Read the model definition and answer for the solid it produces. Units are mm, in the model's axes. Give positions to 0.01 mm unless a question says otherwise; leave off trailing zeros. Order: outer loops, then holes, each group sorted by start corner. A loop starts at its lowest first (then second) coordinate and runs counter-clockwise, first axis right, second up.
```python
from build123d import *

# Parameters (mm, degrees)
SKETCH1_R           = 80.645
BOSS_EXTRUDE1_DEPTH = 7.9375
SKETCH3_R           = 31.877
CUT_EXTRUDE1_DEPTH  = 16.875
CHAMFER1_SIZE       = 3.175
SKETCH5_R           = 5.7546875
CUT_EXTRUDE2_DEPTH  = 16.875
CIRPATTERN1_COUNT   = 5
SKETCH6_R           = 5.7546875
CUT_EXTRUDE3_DEPTH  = 16.875
CIRPATTERN2_COUNT   = 5


with BuildPart() as part:
    # Sketch1 → Boss-Extrude1 (new body, symmetric)
    with BuildSketch(Plane(origin=(0, 0, 0), x_dir=(0, 0, -1), z_dir=(1, 0, 0))):
        Circle(SKETCH1_R)
    extrude(amount=BOSS_EXTRUDE1_DEPTH, both=True)

    # Sketch3 → Cut-Extrude1 (cut, through all)
    with BuildSketch(Plane(origin=(7.9375, 0, 0), x_dir=(0, 0, -1), z_dir=(1, 0, 0))):
        Circle(SKETCH3_R)
    extrude(amount=-CUT_EXTRUDE1_DEPTH, mode=Mode.SUBTRACT)

    # Chamfer1
    chamfer1_edges = [part.edges().sort_by_distance(p)[0] for p in [
        (-7.9375, 0, 31.877),
        (7.9375, 0, 31.877),
    ]]
    chamfer(chamfer1_edges, length=CHAMFER1_SIZE)

    # Sketch5 → Cut-Extrude2 (cut, through all)
    with BuildSketch(Plane(origin=(7.9375, 0, 0), x_dir=(0, 0, -1), z_dir=(1, 0, 0))):
        with Locations((0, 57.15)):
            Circle(SKETCH5_R)
    cut_extrude2 = extrude(amount=-CUT_EXTRUDE2_DEPTH, mode=Mode.SUBTRACT)

    # CirPattern1: Cut-Extrude2 ×5 about axis
    cirpattern1_axis = Axis((0, 0, 0), (1, 0, 0))
    for i in range(1, CIRPATTERN1_COUNT):
        add(cut_extrude2.rotate(cirpattern1_axis, i * 360 / CIRPATTERN1_COUNT), mode=Mode.SUBTRACT)

    # Sketch6 → Cut-Extrude3 (cut, through all)
    with BuildSketch(Plane(origin=(7.9375, 0, 0), x_dir=(0, 0, -1), z_dir=(1, 0, 0))):
        with Locations((0, -57.15)):
            Circle(SKETCH6_R)
    cut_extrude3 = extrude(amount=-CUT_EXTRUDE3_DEPTH, mode=Mode.SUBTRACT)

    # CirPattern2: Cut-Extrude3 ×5 about axis
    cirpattern2_axis = Axis((0, 0, 0), (1, 0, 0))
    for i in range(1, CIRPATTERN2_COUNT):
        add(cut_extrude3.rotate(cirpattern2_axis, i * 360 / CIRPATTERN2_COUNT), mode=Mode.SUBTRACT)


solid = part.part
```
1) Consider L1, parallel to Y at x = -1, z = 0 (3 decimals); L2, parallel to Y at x = 7.25, z = -3; L3, parallel to Y at x = 4.5, z = -37. Determine where each line is inside the solid, lowest interval first.
Final values:
L1: y = -80.645 to -62.905, -51.395 to -31.877, 31.877 to 51.395, 62.905 to 80.645
L2: y = -80.59 to -62.06, -52.24 to -34.23, 34.23 to 52.24, 62.06 to 80.59
L3: y = -71.66 to -50.87, -41.6 to 41.6, 50.87 to 71.66
2) For a pull along Y with two mould halves and no side action, classify faces 1 (the face through (0.067, 9.575, -30.405)), 2 (the face through (0.11, 24.22, -76.92)), 3 (the face through (-7.938, -17, -35)), 4 (the face through (0.111, 22.896, -56.741)) as released by +Y, released by -Y, zero draft, split by the parting line, or undercut.
Final values:
face 1: undercut
face 2: split by the parting line
face 3: zero draft
face 4: undercut
3) The part is cut by section B-B on z = 0. Determine the outline of the cut face in (x, y) (1 decimal), and give its area (3 significant figures).
Final values:
outline: (-7.9, -80.6) - (7.9, -80.6) - (7.9, -62.9) - (-7.9, -62.9) - close; (-7.9, -51.4) - (7.9, -51.4) - (7.9, -35.1) - (4.8, -31.9) - (-4.8, -31.9) - (-7.9, -35.1) - close; (-7.9, 35.1) - (-4.8, 31.9) - (4.8, 31.9) - (7.9, 35.1) - (7.9, 51.4) - (-7.9, 51.4) - close; (-7.9, 62.9) - (7.9, 62.9) - (7.9, 80.6) - (-7.9, 80.6) - close
area: 1,160 mm2
4) The part is cut by section C-C on z = 58. Determine the outline of the cut face in (x, y).
Final values:
outline: (-7.94, -56.03) - (7.94, -56.03) - (7.94, -22.11) - (-7.94, -22.11) - close; (-7.94, -13.21) - (7.94, -13.21) - (7.94, 13.21) - (-7.94, 13.21) - close; (-7.94, 22.11) - (7.94, 22.11) - (7.94, 56.03) - (-7.94, 56.03) - close
5) The part is cut by section A-A on y = 0. Determine the outline of the cut face in (x, z) (1 decimal), and give its area (3 significant figures).
Final values:
outline: (-7.9, -80.6) - (7.9, -80.6) - (7.9, -35.1) - (4.8, -31.9) - (-4.8, -31.9) - (-7.9, -35.1) - close; (-7.9, 35.1) - (-4.8, 31.9) - (4.8, 31.9) - (7.9, 35.1) - (7.9, 80.6) - (-7.9, 80.6) - close
area: 1,530 mm2
6) Given pin 1 (10.5 mm diameter, centred on y = 46.24, z = -33.59, fed in from +X); pin 2 (6 mm diameter, centred on x = -0.5, y = -50, fed in from +Z); pin 3 (2 mm diameter, centred on x = 1.5, y = 47, fed in from +Z); pin 4 (8 mm diameter, centred on x = -0.5, y = -15, fed in from +Z), each flat-ended and moving along its own axis, determine where each tip first touches the part or whether it passes through.
Final values:
pin 1: passes through
pin 2: stops at z = 65.53
pin 3: stops at z = 66.24
pin 4: stops at z = 79.89
7) The part is cut by section D-D on y = -57.15. Determine the outline of the cut face in (x, z).
Final values:
outline: (-7.94, -56.9) - (7.94, -56.9) - (7.94, -5.75) - (-7.94, -5.75) - close; (-7.94, 5.75) - (7.94, 5.75) - (7.94, 56.9) - (-7.94, 56.9) - close
